Autodesk Inventor part; units mm, degrees
ref_plane "YZ Plane" through (0, 0, 0) normal (1, 0, 0) x (0, 1, 0)
ref_plane "XZ Plane" through (0, 0, 0) normal (0, 1, 0) x (-1, 0, 0)
ref_plane "XY Plane" through (0, 0, 0) normal (0, 0, 1) x (1, 0, 0)
sketch "Sketch1" plane through (0, 0, 0) normal (1, 0, 0) x (0, 1, 0)
  line L0 (0, 0) -> (0, -88.9)
  line L1 (0, -88.9) -> (-63.5, -88.9)
  line L2 (-63.5, -88.9) -> (-63.5, 0)
  line L3 (-63.5, 0) -> (0, 0)
  dimension "d0" = 88.9
  dimension "d1" = 63.5
extrude "Extrusion1" add sketch "Sketch1" along normal blind 25.4
sketch "Sketch2" plane through (25.4, 0, 0) normal (1, 0, 0) x (0, 0, -1)
  point P0 (0, 0)
sketch "Sketch3" plane through (25.4, 0, 0) normal (1, 0, 0) x (0, 0, -1)
  line L0 (0, 0) -> (0, -63.5)
  line L1 (0, -25.4) -> (38.1, -25.4)
  line L2 (38.1, -25.4) -> (38.1, -38.1)
  line L3 (38.1, -38.1) -> (0, -38.1)
  line L4 (0, -25.4) -> (0, -38.1)
  dimension "d4" = 25.4
  dimension "d5" = 38.1
  dimension "d6" = 12.7
extrude "Extrusion2" cut sketch "Sketch3" against normal blind 25.4
sketch "Sketch4" plane through (25.4, 0, 0) normal (1, 0, 0) x (0, 0, -1)
  line L0 (0, 0) -> (88.9, 0)
  line L1 (88.9, 0) -> (63.5, 0)
  line L2 (63.5, 0) -> (63.5, -63.5)
  line L3 (0, -63.5) -> (88.9, -63.5)
  line L4 (63.5, -63.5) -> (88.9, -63.5)
  line L5 (88.9, -63.5) -> (88.9, 0)
  dimension "d9" = 25.4
extrude "Extrusion3" add sketch "Sketch4" along normal blind 38.1
sketch "Sketch5" plane through (63.5, 0, 0) normal (1, 0, 0) x (0, 0, -1)
  point P0 (0, 0)
sketch "Sketch6" plane through (63.5, 0, 0) normal (1, 0, 0) x (0, 0, -1)
  line L0 (63.5, -12.7) -> (88.9, -12.7)
  line L1 (88.9, -12.7) -> (88.9, -50.8)
  line L2 (88.9, -63.5) -> (88.9, 0)
  line L3 (88.9, -50.8) -> (63.5, -50.8)
  line L4 (63.5, -63.5) -> (63.5, 0)
  line L5 (63.5, -12.7) -> (63.5, -50.8)
  point P0 (0, 0)
  dimension "d12" = 12.7
  dimension "d13" = 38.1
extrude "Extrusion4" cut sketch "Sketch6" against normal blind 12.7
properties part number "Model Creation 3"
Check sheet for the modelled part. Datum: model origin and axes. Units: mm. A direction names the side the tool comes from. Round coordinates to 2 decimals unless told otherwise and drop trailing zeros. Order: outer loops, then holes, each group sorted by start corner. A loop starts at its lowest first (then second) coordinate and runs counter-clockwise, first axis right, second up.
1) Section check C-C (x = 6). Record the boundary of the cut face in (y, z), and give its area (3 significant figures).
2) Section check A-A (x = 57). Record the boundary of the cut face in (y, z).
3) Section check D-D (y = -16). Record the boundary of the cut face in (x, z), and give its area (3 significant figures).
4) Mould release check, pull along Y, two halves, no side actions. Record for faces 1 (the flat face through (63.5, -6, -76)), 2 (the flat face through (13, -32, -38.1)), 3 (the flat face through (24, 0, -54)), 4 (the flat face through (50.8, -31, -76)): +Y half, -Y half, draft (parallel to the pull), parting line (faces both ways), or undercut.
5) Scan lines: line 1 (Y direction, x = 56, z = -85); line 2 (Y direction, x = 14.5, z = -28.5); line 3 (X direction, y = -9.5, z = -8.5). Record each from-to range of solid material in increasing order.
6) Section check B-B (z = -66.5). Record the boundary of the cut face in (x, y), and give its area (3 significant figures).
7) Go/stop test with flat-tipped pins: pin 1 Ø19 at (y, z) = (-38.5, -35) entering from +X; pin 2 Ø19 at (x, y) = (39, -36.5) entering from +Z; pin 3 Ø4 at (x, y) = (13.5, -33.5) entering from +Z. Record where each tip stops, or that it passes through.
8) Tool access check on faces 5 (the flat face through (13, -25.4, -19)), 6 (the flat face through (25.4, -32.2, -38.4)), 7 (the flat face through (57, -12.7, -76)). Record the directions out of +Z, -Z, +X, -X, +Y, -Y that give a thin tool (end or side, any length) a straight path to the whole face; none if there is none.
Result:
1. outline: (-63.5, -88.9) - (0, -88.9) - (0, 0) - (-25.4, 0) - (-25.4, -38.1) - (-38.1, -38.1) - (-38.1, 0) - (-63.5, 0) - close
1. area: 5,160 mm2
2. outline: (-63.5, -88.9) - (-50.8, -88.9) - (-50.8, -63.5) - (-63.5, -63.5) - close; (-12.7, -88.9) - (0, -88.9) - (0, -63.5) - (-12.7, -63.5) - close
3. outline: (0, -88.9) - (50.8, -88.9) - (50.8, -63.5) - (25.4, -63.5) - (25.4, 0) - (0, 0) - close
3. area: 2,900 mm2
4. face 1: draft
4. face 2: undercut
4. face 3: +Y half
4. face 4: undercut
5. line 1: y = -63.5 to -50.8, -12.7 to 0
5. line 2: y = -63.5 to -38.1, -25.4 to 0
5. line 3: x = 0 to 25.4
6. outline: (0, -63.5) - (63.5, -63.5) - (63.5, -50.8) - (50.8, -50.8) - (50.8, -12.7) - (63.5, -12.7) - (63.5, 0) - (0, 0) - close
6. area: 3,550 mm2
7. pin 1: stops at x = 25.4
7. pin 2: stops at z = -63.5
7. pin 3: stops at z = -38.1
8. face 5: +Z, +X, -X
8. face 6: +Z, +X, +Y, -Y
8. face 7: +Z, -Z, +X
